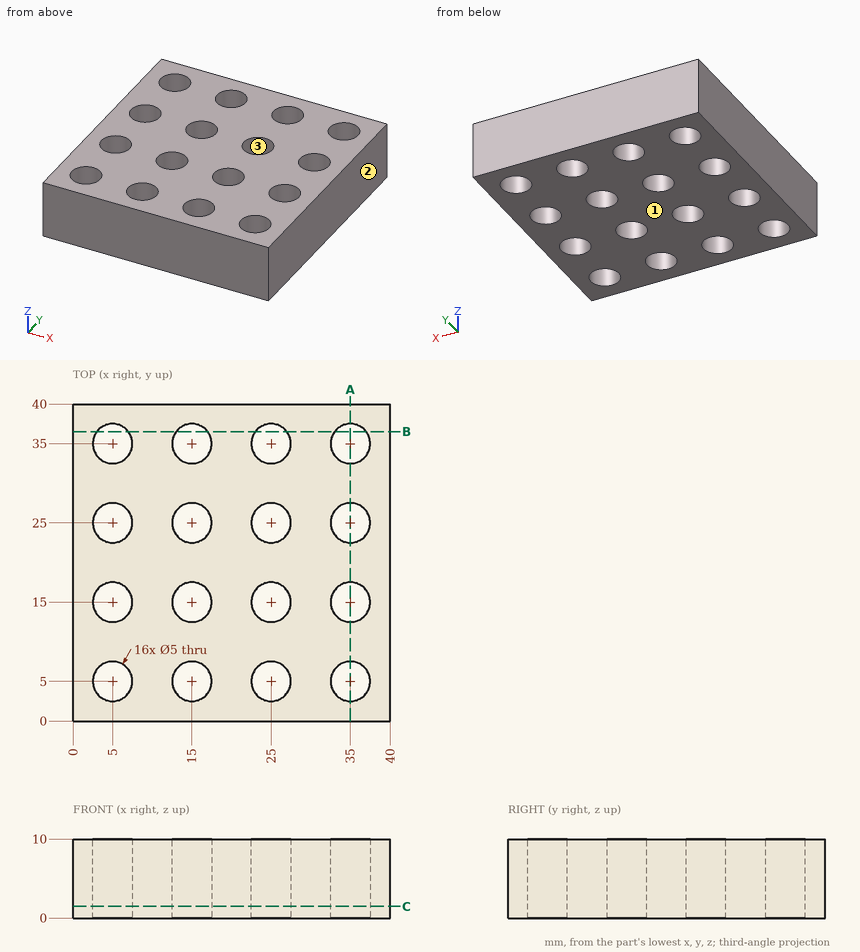
Answer from the drawing. Dimensions are ordinates in mm from the lowest x, y and z of the part. Coordinates: 2 decimals unless noted, no trailing zeros. Loops run counter-clockwise (first coordinate to the right, second up) from the corner with the lowest first, then second, coordinate; pieces in that order, holes last. Notation, with made-up numbers: (-27.5, 4) -> (5.5, 4) arc R4 ccw to (5.5, 8) -> close; hole circle Ø2 at (50, -23.5). An arc over 180 degrees is marked (long way). Answer in a Markdown table with one row per item.
Item 1: A cutting plane is placed at B-B on y = 36.5. Determine the outline of the cut face in (x, z).
Returned:
| item | result |
|---|---|
| outline | (0, 0) -> (3, 0) -> (3, 10) -> (0, 10) -> close; (7, 0) -> (13, 0) -> (13, 10) -> (7, 10) -> close; (17, 0) -> (23, 0) -> (23, 10) -> (17, 10) -> close; (27, 0) -> (33, 0) -> (33, 10) -> (27, 10) -> close; (37, 0) -> (40, 0) -> (40, 10) -> (37, 10) -> close |
Item 2: For a pull along X with two mould halves and no side action, classify the marked faces 1, 2 and 3 as released by +X, released by -X, zero draft, split by the parting line, or undercut.
Returned:
| item | result |
|---|---|
| face 1 | zero draft |
| face 2 | released by +X |
| face 3 | undercut |
Item 3: A cutting plane is placed at C-C on z = 1.5. Give the number of separate pieces and of enclosed holes in the cut face, plus the area to 3 significant figures.
Returned:
| item | result |
|---|---|
| separate pieces | 1 |
| enclosed holes | 16 |
| area | 1,290 mm^2 |
Item 4: This flat-tipped pin is pushed along its axis until it touches: P1, Ø3, axis at x = 15, y = 15, coming from the +Z side. Where does it stop, or does it pass through?
Returned:
| item | result |
|---|---|
| P1 | passes through |
Item 5: A cutting plane is placed at A-A on x = 35. Determine the outline of the cut face in (y, z), plus the area to 3 significant figures.
Returned:
| item | result |
|---|---|
| outline | (0, 0) -> (2.5, 0) -> (2.5, 10) -> (0, 10) -> close; (7.5, 0) -> (12.5, 0) -> (12.5, 10) -> (7.5, 10) -> close; (17.5, 0) -> (22.5, 0) -> (22.5, 10) -> (17.5, 10) -> close; (27.5, 0) -> (32.5, 0) -> (32.5, 10) -> (27.5, 10) -> close; (37.5, 0) -> (40, 0) -> (40, 10) -> (37.5, 10) -> close |
| area | 200 mm^2 |
Item 6: Straight lines are drawn through the part: line 1 along Y through (x, z) = (35, 5); line 2 along Y through (x, z) = (3.5, 4.75). For each, find the intervals that lie inside material, in ascending order. Write a range as [from, to].
Returned:
| item | result |
|---|---|
| line 1 | y = [0, 2.5], [7.5, 12.5], [17.5, 22.5], [27.5, 32.5], [37.5, 40] |
| line 2 | y = [0, 3], [7, 13], [17, 23], [27, 33], [37, 40] |
